from build123d import *

# Parameters (mm, degrees)
SKETCH1_R           = 73.66
BOSS_EXTRUDE1_DEPTH = 7.62
SKETCH2_R           = 3.175
BOSS_EXTRUDE2_DEPTH = 63.5
SKETCH3_R           = 73.66
BOSS_EXTRUDE3_DEPTH = 7.62


with BuildPart() as part:
    # Sketch1 → Boss-Extrude1 (new body)
    with BuildSketch(Plane(origin=(0, 0, 0), x_dir=(1, 0, 0), z_dir=(0, 1, 0))):
        with Locations(Location((0, 0, 0), (0, 0, 90))):
            Circle(SKETCH1_R)
    extrude(amount=BOSS_EXTRUDE1_DEPTH)

    # Sketch2 → Boss-Extrude2 (add)
    with BuildSketch(Plane(origin=(0, 7.62, 0), x_dir=(1, 0, 0), z_dir=(0, 1, 0))):
        with Locations(Location((0, 46, 0), (0, 0, 270))):
            Circle(SKETCH2_R)
        with Locations(Location((0, -46, 0), (0, 0, 270))):
            Circle(SKETCH2_R)
    boss_extrude2 = extrude(amount=BOSS_EXTRUDE2_DEPTH)

    # Mirror1: Boss-Extrude2 across plane
    add(boss_extrude2.mirror(Plane.ZX.offset(71.12)))

    # Sketch3 → Boss-Extrude3 (add)
    with BuildSketch(Plane(origin=(0, 134.62, 0), x_dir=(1, 0, 0), z_dir=(0, 1, 0))):
        with Locations(Location((0, 0, 0), (0, 0, 90))):
            Circle(SKETCH3_R)
    extrude(amount=BOSS_EXTRUDE3_DEPTH)


solid = part.part
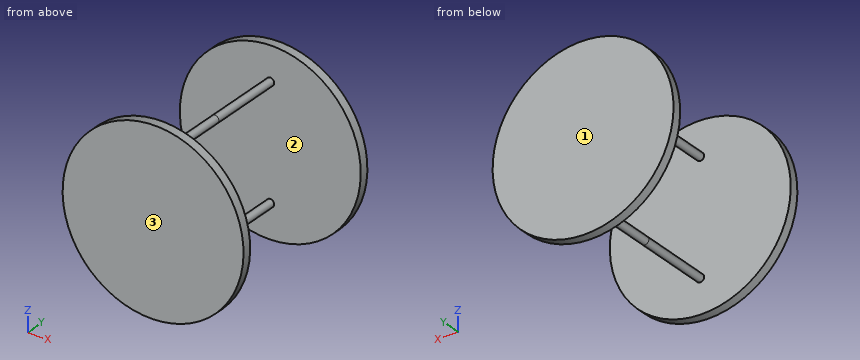
CAD build for the part. Positions are in the model's coordinates, mm. Face numbers are marked on the shaded views. Round coordinates to 2 decimals unless told otherwise and drop trailing zeros. Order: outer loops, then holes, each group sorted by start corner. A loop starts at its lowest first (then second) coordinate and runs counter-clockwise, first axis right, second up. Notation, with made-up numbers: (45, -14) - (79, -14) arc R30 cw to (79, 18) - close; hole circle Ø9 at (1, -18). An arc over 180 degrees is marked (long way). Return JSON: item names as keys, results as strings.
(1) Cut at B-B (x = -10.5). Give the cut face in (y, z).
Answer key:
{"outline": "(0, -72.91) - (7.62, -72.91) - (7.62, 72.91) - (0, 72.91) - close; (134.62, -72.91) - (142.24, -72.91) - (142.24, 72.91) - (134.62, 72.91) - close"}
(2) Cut at A-A (z = 0). Give the cut face in (x, y).
Answer key:
{"outline": "(-73.66, 0) - (73.66, 0) - (73.66, 7.62) - (-73.66, 7.62) - close; (-73.66, 134.62) - (73.66, 134.62) - (73.66, 142.24) - (-73.66, 142.24) - close"}
(3) Pin check, flat tips, straight feed: pin 1 Ø12 at (x, y) = (-2.5, 41) entering from -Z (3 decimals); pin 2 Ø10 at (y, z) = (51.5, 45) entering from +X (3 decimals). Stop position of each tip, or through.
Answer key:
{"pin 1": "stops at z = -49.175", "pin 2": "stops at x = 3.175"}
(4) Cut at C-C (y = 14). Give the cut face in (x, z) (3 decimals).
Answer key:
{"outline": "circle Ø6.35 at (0, -46); circle Ø6.35 at (0, 46)"}
(5) Wall check: probe 1 along Y at (x, z) = (-58, -7.5). Give the ranges that are in metal, low to high. Write a range as from..to.
Answer key:
{"probe 1": "y = 0..7.62, 134.62..142.24"}
(6) Pull direction Y, two halves, no side cores. Call the marked faces 1, 2 and 3: +Y half, -Y half, draft (parallel to the pull), parting line (faces both ways), or undercut.
Answer key:
{"face 1": "+Y half", "face 2": "undercut", "face 3": "-Y half"}
(7) Cut at D-D (z = -46). Give the cut face in (x, y) (3 decimals), then the cut area to 3 significant figures.
Answer key:
{"outline": "(-57.531, 0) - (57.531, 0) - (57.531, 7.62) - (3.175, 7.62) - (3.175, 134.62) - (57.531, 134.62) - (57.531, 142.24) - (-57.531, 142.24) - (-57.531, 134.62) - (-3.175, 134.62) - (-3.175, 7.62) - (-57.531, 7.62) - close", "area": "2,560 mm^2"}
